CAD build for the part. Positions are in the model's coordinates, mm. A direction names the side the tool comes from. Coordinates: 2 decimals unless noted, no trailing zeros. Return JSON: item names as keys, results as strings.
from build123d import *

# Parameters (mm, degrees)
F2_DEPTH = 2.5
F3_DEPTH = 2.5
F4_SIZE  = 2.49999
F8_DEPTH = 2.5
F9_SIZE  = 2.49999
F10_D    = 2.5


# Not quite as in the source:
# - a fillet or chamfer is up to 0.001 mm smaller than in the source, because OpenCascade refuses the exact size
# - a feature of the source that left no trace in its solid (it failed there, or was rolled back) is left out


with BuildPart() as f2:
    # F0 (on Front) → F2 (new body)
    with BuildSketch(Plane.XZ):
        Polygon((0, 7.5), (-15, 7.5), (-15, 2.5), (-5, 2.5), (-5, -2.5), (-15, -2.5), (-15, -7.5), (0, -7.5), align=None)
    extrude(amount=-F2_DEPTH)

    # F1 (on Right) → F3 (join)
    with BuildSketch(Plane.YZ):
        Polygon((15, -7.5), (15, -2.4617532641), (15, 5), (15, 7.5), (10, 7.5), (10, 5), (10, -2.4617532641), (0, -2.4617532641), (0, -7.5), align=None)
    extrude(amount=-F3_DEPTH)

    # F4 (call 1 of 3: OpenCascade refuses the feature's edges together) (size 2.5 in the source; OpenCascade refuses exactly that, so slightly less here)
    f4_edges = [f2.edges().sort_by_distance(p)[0] for p in [
        (0, 2.5, 2.519123),
    ]]
    chamfer(f4_edges, length=F4_SIZE)

    # F4#2 (call 2 of 3) (size 2.5 in the source; OpenCascade refuses exactly that, so slightly less here)
    f4_2_edges = [f2.edges().sort_by_distance(p)[0] for p in [
        (-10, 2.5, -2.5),
    ]]
    chamfer(f4_2_edges, length=F4_SIZE)

    # F4#3 (call 3 of 3) (size 2.5 in the source; OpenCascade refuses exactly that, so slightly less here)
    f4_3_edges = [f2.edges().sort_by_distance(p)[0] for p in [
        (-2.5, 10, 2.519123),
        (-2.5, 6.25, -2.461753),
    ]]
    chamfer(f4_3_edges, length=F4_SIZE)

    # F7 (on offset) → F8 (join)
    with BuildSketch(Plane.XY.offset(7.5)):
        Polygon((0, 0), (0, 15), (-5, 15), (-5, 5), (-10, 5), (-10, 15), (-15, 15), (-15, 0), align=None)
    extrude(amount=-F8_DEPTH)

    # F9 (size 2.5 in the source; OpenCascade refuses exactly that, so slightly less here)
    f9_edges = [f2.edges().sort_by_distance(p)[0] for p in [
        (-10, 10, 5),
    ]]
    chamfer(f9_edges, length=F9_SIZE)

    # F10 (through all)
    with Locations(Plane.XY.offset(7.5)):
        with Locations((-12.5, 12.5)):
            Hole(F10_D / 2)


solid = f2.part
Item 1: Which spindle directions (+Z, -Z, +X, -X, +Y, -Y) get a long thin tool onto all of the face, cutting with end or side? Do faces 1 (the flat face through (-1, 11, 1)), 2 (the flat face through (-8, 5, 6)), 3 (the flat face through (-9.9, 1.3, -3.8)), 4 (the flat face through (-1.27, 6.34, -3.73)). Say none if no direction does.
Findings below:
{"face 1": "-X", "face 2": "-Z, +Y", "face 3": "-X, +Y", "face 4": "none"}
Item 2: Wall check: L1, parallel to X at y = 12.5, z = 6.8; L2, parallel to Y at x = -12.5, z = 6.3; L3, parallel to X at y = 12.5, z = 5.85. Give the ranges that are in metal, low to high. Write a range as [from, to].
Findings below:
{"L1": "x = [-15, -13.75], [-11.25, -10.7], [-5, 0]", "L2": "y = [0, 11.25], [13.75, 15]", "L3": "x = [-15, -13.75], [-5, 0]"}
Item 3: Mould opens along X. For faces 5 (the flat face through (-8, 4, 7.5)), 6 (the flat face through (-11.3, 9.9, 6.2)), 7 (the flat face through (0, 11, 0)) say: released by +X, released by -X, zero draft, split by the parting line, or undercut.
Findings below:
{"face 5": "zero draft", "face 6": "undercut", "face 7": "released by +X"}
Item 4: Drop flat-ended pins along their axis: P1, Ø1.2, axis at y = 1.5, z = -0.5, coming from the -X side; P2, Ø3, axis at x = -11, y = 5.5, coming from the -Z side; P3, Ø3, axis at x = -8, z = 6.5, coming from the +Y side. Give the stop position or say it passes through.
Findings below:
{"P1": "stops at x = -5", "P2": "stops at z = 5", "P3": "stops at y = 5"}
Item 5: Band-saw the part on B-B, the plane y = 7. Count the separate pieces of the cut face and the enclosed holes in it, then the cut area to 3 significant figures.
Findings below:
{"separate pieces": "3", "enclosed holes": "0", "area": "31.3 mm²"}
